from build123d import *

# Parameters (mm, degrees)
CYLINDER_R        = 6.25
CYLINDER_DEPTH    = 2.5
CYLINDER001_R     = 8
CYLINDER001_DEPTH = 1
FILLET_R          = 0.9


with BuildPart() as cylinder:
    # Cylinder → Cylinder (new body)
    with BuildSketch(Plane.XY):
        Circle(CYLINDER_R)
    extrude(amount=CYLINDER_DEPTH)


with BuildPart() as fillet_body:
    # Cylinder001 → Cylinder001 (new body)
    with BuildSketch(Plane.XY.offset(2.5)):
        Circle(CYLINDER001_R)
    extrude(amount=CYLINDER001_DEPTH)

    # Fusion: union Cylinder
    add(cylinder.part)

    # Fillet
    fillet_edges = [fillet_body.edges().sort_by_distance(p)[0] for p in [
        (-8, 0, 3.5),
    ]]
    fillet(fillet_edges, radius=FILLET_R)


solid = fillet_body.part
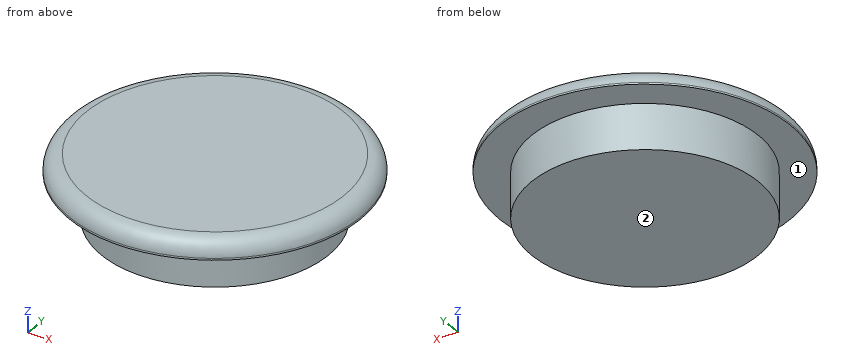
Here's how the part is built. I have some questions about the finished solid (model axes, mm). Face numbers are marked on the shaded views. A direction names the side the tool comes from. Coordinates: 2 decimals unless noted, no trailing zeros. Loops run counter-clockwise (first coordinate to the right, second up) from the corner with the lowest first, then second, coordinate; pieces in that order, holes last. Notation, with made-up numbers: (-12, 80) -> (14, 80) arc R20 ccw to (14, 119) -> close; hole circle Ø4 at (-15.5, 34.25). An arc over 180 degrees is marked (long way). Use one line per item in the form item = value. Start each with the question number.
(1) On a 3-axis mill with a long thin cutter (end or side, diameter ignored), from which of +Z, -Z, +X, -X, +Y, -Y can I reach the whole of each face in a straight line? I mean the marked faces 1 and 2. Say none if no direction works.
(2) Will this pin go through, and if not, where does the flat tip stop? pin 1 (2 mm diameter, centred on x = -1.5, z = 2, fed in from -Y).
(3) If we section it at C-C (z = 0.6): Please give me the cut outline in (x, y), then the cut area to 3 significant figures.
(4) If we section it at A-A (x = 0): Please give me the cut outline in (y, z).
(5) If we section it at D-D (z = 3): Please give me the cut outline in (x, y).
(6) Please list where these lines run through material, in increasing order: line 1 along Z through (x, y) = (-6.25, 2); line 2 along Y through (x, z) = (1.5, 2.9); line 3 along Y through (x, z) = (4.5, 2.8).
Verdict:
q1.face_1 = -Z
q1.face_2 = -Z, +X, -X, +Y, -Y
q2.pin_1 = -7.97
q3.outline = circle Ø12.5 at (0, 0)
q3.area = 123 mm²
q4.outline = (-8, 2.5) -> (-6.25, 2.5) -> (-6.25, 0) -> (6.25, 0) -> (6.25, 2.5) -> (8, 2.5) -> (8, 2.6) arc R0.9 ccw to (7.1, 3.5) -> (-7.1, 3.5) arc R0.9 ccw to (-8, 2.6) -> close
q5.outline = circle Ø15.81 at (0, 0)
q6.line_1 = 2.5 to 3.5
q6.line_2 = -7.81 to 7.81
q6.line_3 = -6.59 to 6.59
